Autodesk Fusion 360 part; units mm, degrees
sketch "Sketch1" plane through (0, 0, 0) normal (0, 0, 1) x (1, 0, 0)
  line L0 (0, 0) -> (20, 0)
  line L1 (20, 0) -> (20, -16)
  line L2 (20, -16) -> (0, -16)
  line L3 (0, -16) -> (0, 0)
  line L4 (20, -8) -> (0, -8) construction
  line L5 (10, 0) -> (10, -16) construction
  line L6 (7.5, -6) -> (7.5, -10)
  arc A0 (7.5, -10) -> (12.5, -10) centre (10, -10) ccw
  line L7 (12.5, -10) -> (12.5, -6)
  arc A1 (12.5, -6) -> (7.5, -6) centre (10, -6) ccw
  line L8 (10, -6) -> (10, -10) construction
  line L9 (5.5, -6) -> (5.5, -10)
  arc A2 (5.5, -10) -> (14.5, -10) centre (10, -10) ccw
  line L10 (14.5, -10) -> (14.5, -6)
  arc A3 (14.5, -6) -> (5.5, -6) centre (10, -6) ccw
  line L11 (10, -6) -> (10, -10) construction
  dimension "d1" = 20
  dimension "d2" = 16
  dimension "d11" = 5
  dimension "d12" = 2
  dimension "d13" = 2
  dimension "d14" = 9
extrude "Extrude1" add sketch "Sketch1" along normal blind 4 contours L0 L1 L2 L3 | L9 A2 L10 A3
extrude "Extrude2" add sketch "Sketch1" along normal blind 5 from surface at 4 contours L0 L1 L2 L3
fillet "Fillet1" radius 2 2 edges at (20, -8, 9) (0, -8, 9)
Work out the finished part from the listing and answer in its coordinate system (mm). A direction names the side the tool comes from. Round coordinates to 2 decimals unless told otherwise and drop trailing zeros. Write each loop counter-clockwise with the first axis right and the second up, starting at its lowest first coordinate (ties: lowest second). Pieces come first, ordered by that corner, then holes. Notation, with made-up numbers: (30.5, 4.25) - (55.5, 4.25) arc R30 cw to (55.5, 28.25) - close; hole circle Ø10 at (58.5, -36.5). An arc over 180 degrees is marked (long way). Return JSON: item names as keys, results as strings. Group by question number.
Q1. For faces 5 (the flat face through (12, -4, 0)), 6 (the cylindrical face through (9.9, -3.5, 2)), 7 (the cylindrical face through (10.1, -14.5, 6.5)), determine the directions among +Z, -Z, +X, -X, +Y, -Y from which every point of the face is accessible in a straight line to the end or side of a thin tool.
Q2. The part is cut by section A-A on z = 4.75. Write down the section's boundary in (x, y).
Q3. The part is cut by section C-C on y = -11.5. Write down the section's boundary in (x, z), then the cut area to 3 significant figures.
Q4. The mould has two halves that part along Y. Classify faces 1 (the flat face through (10, -16, 4)), 2 (the flat face through (15, -8, 9)), 3 (the flat face through (10, 0, 4)), 4 (the cylindrical face through (10.1, -12.5, 2)): released by +Y, released by -Y, zero draft, split by the parting line, or undercut.
Q5. The part is cut by section D-D on z = 1.75. Write down the section's boundary in (x, y).
Q6. Find the intervals of material crossed by L1, parallel to X at y = -7.5, z = 3.5; L2, parallel to X at y = -8.5, z = 6.25; L3, parallel to Z at x = 14, y = -5, in increasing order.
Q7. The part is cut by section B-B on x = 10. Write down the section's boundary in (y, z), then the cut area to 3 significant figures.
Solved:
{
 "1": {"face 5": "-Z, +X, -X, +Y, -Y", "face 6": "+Z, -Z", "face 7": "+Z"},
 "2": {"outline": "(0, -16) - (20, -16) - (20, 0) - (0, 0) - close; hole (5.5, -10) arc R4.5 ccw to (14.5, -10) - (14.5, -6) arc R4.5 ccw to (5.5, -6) - close"},
 "3": {"outline": "(0, 0) - (8, 0) - (8, 4) - (5.76, 4) - (5.76, 9) - (2, 9) arc R2 ccw to (0, 7) - close; (12, 0) - (20, 0) - (20, 7) arc R2 ccw to (18, 9) - (14.24, 9) - (14.24, 4) - (12, 4) - close", "area": "120 mm²"},
 "4": {"face 1": "released by -Y", "face 2": "zero draft", "face 3": "released by +Y", "face 4": "undercut"},
 "5": {"outline": "(0, -16) - (20, -16) - (20, 0) - (0, 0) - close; hole (7.5, -10) arc R2.5 ccw to (12.5, -10) - (12.5, -6) arc R2.5 ccw to (7.5, -6) - close"},
 "6": {"L1": "0 to 7.5, 12.5 to 20", "L2": "0 to 5.5, 14.5 to 20", "L3": "0 to 4"},
 "7": {"outline": "(-16, 0) - (-12.5, 0) - (-12.5, 4) - (-14.5, 4) - (-14.5, 9) - (-16, 9) - close; (-3.5, 0) - (0, 0) - (0, 9) - (-1.5, 9) - (-1.5, 4) - (-3.5, 4) - close", "area": "43.0 mm²"}
}
